For this review, use the dimensioned drawing (mm, ordinates from the lowest corner) and the shaded views. A direction names the side the tool comes from. Round coordinates to 2 decimals unless told otherwise and drop trailing zeros. Order: outer loops, then holes, each group sorted by start corner. A loop starts at its lowest first (then second) coordinate and runs counter-clockwise, first axis right, second up. Notation, with made-up numbers: (-36.5, 30.5) - (-26.5, 30.5) arc R19 ccw to (-26.5, 46.5) - close; hole circle Ø1 at (-27.5, 80.5). An arc over 180 degrees is marked (long way). Write each question's results on one line, items separated by ' | '. Start each with the question number.
(1) Take a section at D-D, the plane z = 2. Give the boundary of the cut face in (x, y).
(2) Take a section at C-C, the plane y = 4.25. Give the boundary of the cut face in (x, z), plus the area to 4 significant figures.
(3) Take a section at A-A, the plane z = 0.5. Give the boundary of the cut face in (x, y).
(4) For L1, parallel to Y at x = 6.25, z = 3.95; L2, parallel to X at y = 6, z = 3.25; L3, parallel to X at y = 3.5, z = 6.5, list the stretches that pass through material, from the lowest coordinate up. Write a range as from..to.
(5) For the marked faces 1, 2 and 3, list the 3-axis set-ups (+Z, -Z, +X, -X, +Y, -Y) from which the entire face can be reached by the end or side of a thin tool; tool diameter is ignored.
(6) Take a section at B-B, the plane x = 6.25. Give the boundary of the cut face in (y, z).
(7) Draft analysis for pull direction X (two halves, no side actions). For the marked faces 4, 5 and 6, state which applies: pulls with the +X half, pulls with the -X half, needs draft (parallel to the pull), parting line crosses it, or undercut.
(8) Insertion check: pin 1 Ø1 at (x, z) = (6, 5.5) entering from +Y; pin 2 Ø2 at (y, z) = (5.5, 4.5) entering from -X; pin 3 Ø0.8 at (x, z) = (5.5, 0.5) entering from -Y. Each pin has a flat end and moves straight along its axis. Give the tip position at first contact, or say it passes through.
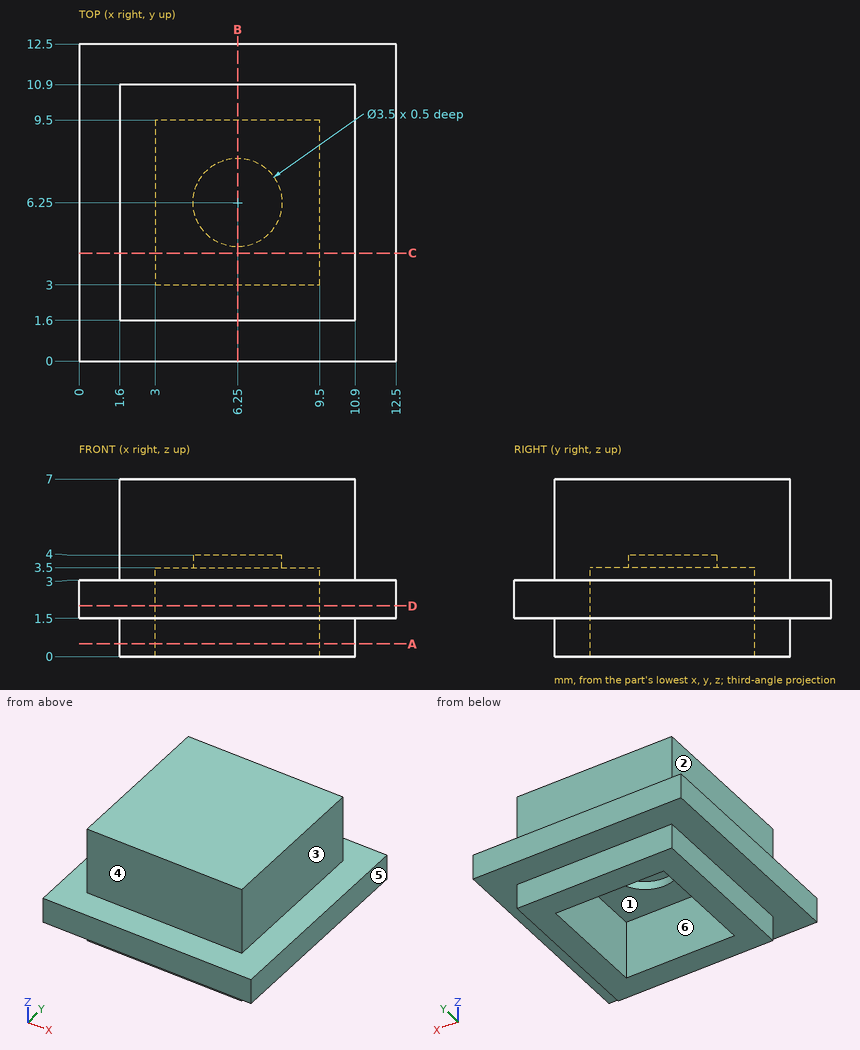
Results below:
1) outline: (0, 0) - (12.5, 0) - (12.5, 12.5) - (0, 12.5) - close; hole (3, 3) - (9.5, 3) - (9.5, 9.5) - (3, 9.5) - close
2) outline: (0, 1.5) - (1.6, 1.5) - (1.6, 0) - (3, 0) - (3, 3.5) - (9.5, 3.5) - (9.5, 0) - (10.9, 0) - (10.9, 1.5) - (12.5, 1.5) - (12.5, 3) - (10.9, 3) - (10.9, 7) - (1.6, 7) - (1.6, 3) - (0, 3) - close | area: 47.15 mm^2
3) outline: (1.6, 1.6) - (10.9, 1.6) - (10.9, 10.9) - (1.6, 10.9) - close; hole (3, 3) - (9.5, 3) - (9.5, 9.5) - (3, 9.5) - close
4) L1: y = 1.6..4.5, 8..10.9 | L2: x = 1.6..3, 9.5..10.9 | L3: x = 1.6..10.9
5) face 1: -Z | face 2: +Z, -X, +Y, -Y | face 3: +Z, +X, +Y, -Y
6) outline: (0, 1.5) - (1.6, 1.5) - (1.6, 0) - (3, 0) - (3, 3.5) - (4.5, 3.5) - (4.5, 4) - (8, 4) - (8, 3.5) - (9.5, 3.5) - (9.5, 0) - (10.9, 0) - (10.9, 1.5) - (12.5, 1.5) - (12.5, 3) - (10.9, 3) - (10.9, 7) - (1.6, 7) - (1.6, 3) - (0, 3) - close
7) face 4: needs draft | face 5: pulls with the +X half | face 6: undercut
8) pin 1: stops at y = 10.9 | pin 2: stops at x = 1.6 | pin 3: stops at y = 1.6
